Autodesk Inventor part; units mm, degrees
ref_plane "dummy_XY" through (0, 0, 0) normal (0, 0, 1) x (1, 0, 0)
ref_plane "dummy_YZ" through (0, 0, 0) normal (1, 0, 0) x (0, 1, 0)
ref_plane "dummy_ZX" through (0, 0, 0) normal (0, 1, 0) x (0, 0, 1)
sketch "Sketch_1" plane through (0, 0, 0) normal (0, 0, 1) x (1, 0, 0)
  line L0 (-6.35, 6.35) -> (-6.35, -6.35)
  line L1 (-6.35, -6.35) -> (23.8252, -6.35)
  line L2 (23.8252, -6.35) -> (23.8252, 6.35)
  line L3 (23.8252, 6.35) -> (-6.35, 6.35)
extrude "Extrusion1" add sketch "Sketch_1" along normal mid plane 12.7
sketch "Sketch_2" plane through (0, 0, 0) normal (0, 1, 0) x (-1, 0, 0)
  line L0 (6.35, -3.3338) -> (6.35, 3.3338)
  line L1 (6.35, 3.3338) -> (-11.1252, 3.3338)
  line L2 (-11.1252, 3.3338) -> (-11.1252, -3.3338)
  line L3 (-11.1252, -3.3338) -> (6.35, -3.3338)
extrude "Extrusion2" cut sketch "Sketch_2" along normal mid plane 12.7
sketch "Sketch3" plane through (23.8252, -6.35, 6.35) normal (1, 0, 0) x (0, 0, -1)
  point P0 (6.35, 6.35)
hole "Hole1" at (23.8252, 0, 0) direction (-1, 0, 0) diameter 6.7818 depth 11.176 countersink diameter 7.9375 countersink angle 90
sketch "Sketch4" plane through (12.6492, 0, 0) normal (1, 0, 0) x (0, 0, -1)
  point P0 (0, 0)
hole "Hole2" at (12.6492, 0, 0) direction (-1, 0, 0) diameter 6.792 depth 1.524
sketch "Sketch_5" plane through (0, 0, 0) normal (1, 0, 0) x (0, 1, 0)
  line L0 (0, -6.35) -> (0, 6.35)
  line L1 (0, 6.35) -> (4.3371, 6.35)
  line L2 (4.3371, 6.35) -> (3.194, 5.207)
  line L3 (3.194, 5.207) -> (3.194, -5.207)
  line L4 (3.194, -5.207) -> (4.3371, -6.35)
  line L5 (4.3371, -6.35) -> (0, -6.35)
  line L6 (0, -6.35) -> (0, 6.35)
revolve "Revolution1" cut sketch "Sketch_5" angle 360 about axis through (0, 0, -6.35) along (0, 0, -1)
sketch "Sketch_9" plane through (0, 0, 0) normal (0, 0, 1) x (1, 0, 0)
  line L0 (30.1752, 0) -> (23.8252, 0)
  line L1 (23.8252, 0) -> (23.8252, 6.35)
  arc A0 (23.8252, 6.35) -> (21.2852, 12.7) centre (6.6802, 3.175) ccw
  line L2 (21.2852, 12.7) -> (30.1752, 12.7)
  line L3 (30.1752, 12.7) -> (30.1752, 0)
  line L4 (30.1752, 0) -> (23.8252, 0)
revolve "Revolution2" cut sketch "Sketch_9" angle 360 about axis through (30.1752, 0, 0) along (1, 0, 0)
sketch "Sketch_10" plane through (0, 0, 0) normal (0, 0, 1) x (1, 0, 0)
  line L0 (-6.35, 0) -> (-12.7, 0)
  line L1 (-12.7, 0) -> (-12.7, 12.7)
  line L2 (-12.7, 12.7) -> (-3.81, 12.7)
  arc A0 (-3.81, 12.7) -> (-6.35, 6.35) centre (10.795, 3.175) ccw
  line L3 (-6.35, 6.35) -> (-6.35, 0)
  line L4 (-6.35, 0) -> (-12.7, 0)
revolve "Revolution3" cut sketch "Sketch_10" angle 360 about axis through (-6.35, 0, 0) along (1, 0, 0)
ref_plane "dummy_XY" through (0, 0, 0) normal (0, 0, 1) x (1, 0, 0)
ref_plane "dummy_YZ" through (0, 0, 0) normal (1, 0, 0) x (0, 1, 0)
ref_plane "dummy_ZX" through (0, 0, 0) normal (0, 1, 0) x (0, 0, 1)
ref_plane "h1_XY" through (-6.35, 6.35, 0) normal (0, 0, 1) x (1, 0, 0)
ref_plane "h1_YZ" through (-6.35, 6.35, 0) normal (1, 0, 0) x (0, 1, 0)
ref_plane "h1_ZX" through (-6.35, 6.35, 0) normal (0, 1, 0) x (0, 0, 1)
ref_plane "h2_XY" through (-6.35, -6.35, 0) normal (0, 0, 1) x (1, 0, 0)
ref_plane "h2_YZ" through (-6.35, -6.35, 0) normal (1, 0, 0) x (0, 1, 0)
ref_plane "h2_ZX" through (-6.35, -6.35, 0) normal (0, 1, 0) x (0, 0, 1)
ref_plane "l1_XY" through (23.8252, 6.35, 0) normal (0, 0, 1) x (1, 0, 0)
ref_plane "l1_YZ" through (23.8252, 6.35, 0) normal (1, 0, 0) x (0, 1, 0)
ref_plane "l1_ZX" through (23.8252, 6.35, 0) normal (0, 1, 0) x (0, 0, 1)
ref_plane "l11_XY" through (23.8252, 6.35, 0) normal (0, 0, 1) x (1, 0, 0)
ref_plane "l11_YZ" through (23.8252, 6.35, 0) normal (1, 0, 0) x (0, 1, 0)
ref_plane "l11_ZX" through (23.8252, 6.35, 0) normal (0, 1, 0) x (0, 0, 1)
ref_plane "l12_XY" through (0, 6.35, 0) normal (0, 0, 1) x (1, 0, 0)
ref_plane "l12_YZ" through (0, 6.35, 0) normal (1, 0, 0) x (0, 1, 0)
ref_plane "l12_ZX" through (0, 6.35, 0) normal (0, 1, 0) x (0, 0, 1)
ref_plane "l2_XY" through (-6.35, 6.35, 0) normal (0, 0, 1) x (1, 0, 0)
ref_plane "l2_YZ" through (-6.35, 6.35, 0) normal (1, 0, 0) x (0, 1, 0)
ref_plane "l2_ZX" through (-6.35, 6.35, 0) normal (0, 1, 0) x (0, 0, 1)
ref_plane "l21_XY" through (23.8252, 0, 0) normal (0, 1, 0) x (1, 0, 0)
ref_plane "l21_YZ" through (23.8252, 0, 0) normal (1, 0, 0) x (0, 0, -1)
ref_plane "l21_ZX" through (23.8252, 0, 0) normal (0, 0, -1) x (0, 1, 0)
ref_plane "l22_XY" through (11.1252, 0, 0) normal (0, 1, 0) x (1, 0, 0)
ref_plane "l22_YZ" through (11.1252, 0, 0) normal (1, 0, 0) x (0, 0, -1)
ref_plane "l22_ZX" through (11.1252, 0, 0) normal (0, 0, -1) x (0, 1, 0)
ref_plane "piston_rod_clevis_XY" through (23.8252, 0, 0) normal (1, 0, 0) x (0, 0, -1)
ref_plane "piston_rod_clevis_YZ" through (23.8252, 0, 0) normal (0, 0, -1) x (0, 1, 0)
ref_plane "piston_rod_clevis_ZX" through (23.8252, 0, 0) normal (0, 1, 0) x (1, 0, 0)
ref_plane "rod_clevis_body_XY" through (0, 0, 0) normal (0, 0, 1) x (1, 0, 0)
ref_plane "rod_clevis_body_YZ" through (0, 0, 0) normal (1, 0, 0) x (0, 1, 0)
ref_plane "rod_clevis_body_ZX" through (0, 0, 0) normal (0, 1, 0) x (0, 0, 1)
ref_plane "th1_XY" through (23.8252, 3.9688, 0) normal (0, 0, 1) x (1, 0, 0)
ref_plane "th1_YZ" through (23.8252, 3.9688, 0) normal (1, 0, 0) x (0, 1, 0)
ref_plane "th1_ZX" through (23.8252, 3.9688, 0) normal (0, 1, 0) x (0, 0, 1)
ref_plane "th2_XY" through (23.8252, -3.9688, 0) normal (0, 0, 1) x (1, 0, 0)
ref_plane "th2_YZ" through (23.8252, -3.9688, 0) normal (1, 0, 0) x (0, 1, 0)
ref_plane "th2_ZX" through (23.8252, -3.9688, 0) normal (0, 1, 0) x (0, 0, 1)
ref_plane "to_cylinder_XY" through (11.1252, 0, 0) normal (1, 0, 0) x (0, 0, -1)
ref_plane "to_cylinder_YZ" through (11.1252, 0, 0) normal (0, 0, -1) x (0, 1, 0)
ref_plane "to_cylinder_ZX" through (11.1252, 0, 0) normal (0, 1, 0) x (1, 0, 0)
ref_plane "w1_XY" through (23.8252, 0, -6.35) normal (0, 1, 0) x (1, 0, 0)
ref_plane "w1_YZ" through (23.8252, 0, -6.35) normal (1, 0, 0) x (0, 0, -1)
ref_plane "w1_ZX" through (23.8252, 0, -6.35) normal (0, 0, -1) x (0, 1, 0)
ref_plane "w11_XY" through (-6.35, 0, -3.3338) normal (0, 1, 0) x (1, 0, 0)
ref_plane "w11_YZ" through (-6.35, 0, -3.3338) normal (1, 0, 0) x (0, 0, -1)
ref_plane "w11_ZX" through (-6.35, 0, -3.3338) normal (0, 0, -1) x (0, 1, 0)
ref_plane "w12_XY" through (-6.35, 0, 3.3338) normal (0, 1, 0) x (1, 0, 0)
ref_plane "w12_YZ" through (-6.35, 0, 3.3338) normal (1, 0, 0) x (0, 0, -1)
ref_plane "w12_ZX" through (-6.35, 0, 3.3338) normal (0, 0, -1) x (0, 1, 0)
ref_plane "w2_XY" through (23.8252, 0, 6.35) normal (0, 1, 0) x (1, 0, 0)
ref_plane "w2_YZ" through (23.8252, 0, 6.35) normal (1, 0, 0) x (0, 0, -1)
ref_plane "w2_ZX" through (23.8252, 0, 6.35) normal (0, 0, -1) x (0, 1, 0)
properties part number "D-14059"
Geometry check sheet. Reference: the model listing, model coordinates, mm. A direction names the side the tool comes from. Coordinates: 2 decimals unless noted, no trailing zeros. Order: outer loops, then holes, each group sorted by start corner. A loop starts at its lowest first (then second) coordinate and runs counter-clockwise, first axis right, second up. Notation, with made-up numbers: (77, 3) -> (130, 3) arc R13 cw to (130, 11) -> close; hole circle Ø7 at (-26.75, 36.5). An arc over 180 degrees is marked (long way). Use a Markdown table: item, result. Add a question column.
1. Cross-section at B-B (y = 2.75). Give the number of separate pieces and of enclosed holes in the cut face, and give its area (3 significant figures).
2. Cross-section at A-A (x = 18). Enter the section's corners in (y, z).
3. Material ranges on L1, parallel to Y at x = 21, z = 0; L2, parallel to Z at x = -5, y = -4.5, recorded low to high.
4. Go/stop test with flat-tipped pins: pin 1 Ø4 at (y, z) = (0, 0) entering from -X; pin 2 Ø6.5 at (x, y) = (1, 3) entering from +Z; pin 3 Ø4 at (x, y) = (1, -2) entering from -Z; pin 4 Ø4.5 at (y, z) = (-3, 0.5) entering from -X. Record where each tip stops, or that it passes through.
5. Mould release check, pull along X, two halves, no side actions. Record for faces 3 (the face through (9, 0, -6.35)), 4 (the face through (0.959, 3.047, 4.257)), 5 (the face through (23.825, -3, 3)): pulls with the +X half, pulls with the -X half, needs draft (parallel to the pull), parting line crosses it, or undercut.
6. Set-up check for faces 1 (the face through (12, 6.35, 0)), 2 (the face through (4, 0, 3.334)): record each of +Z, -Z, +X, -X, +Y, -Y from which the full face is reachable in a straight line by a thin tool's end or side.
Filled sheet:
| question | item | result |
|---|---|---|
| 1 | separate pieces | 4 |
| 1 | enclosed holes | 0 |
| 1 | area | 192 mm2 |
| 2 | outline | (-6.35, -6.35) -> (6.35, -6.35) -> (6.35, 6.35) -> (-6.35, 6.35) -> close; hole circle Ø6.78 at (0, 0) |
| 3 | L1 | -6.35 to -3.39, 3.39 to 6.35 |
| 3 | L2 | -6.35 to -3.33, 3.33 to 6.35 |
| 4 | pin 1 | through |
| 4 | pin 2 | z = 6.35 |
| 4 | pin 3 | z = -6.25 |
| 4 | pin 4 | x = 11.13 |
| 5 | face 3 | needs draft |
| 5 | face 4 | undercut |
| 5 | face 5 | pulls with the +X half |
| 6 | face 1 | +Z, -Z, +X, -X, +Y |
| 6 | face 2 | -X, +Y, -Y |
